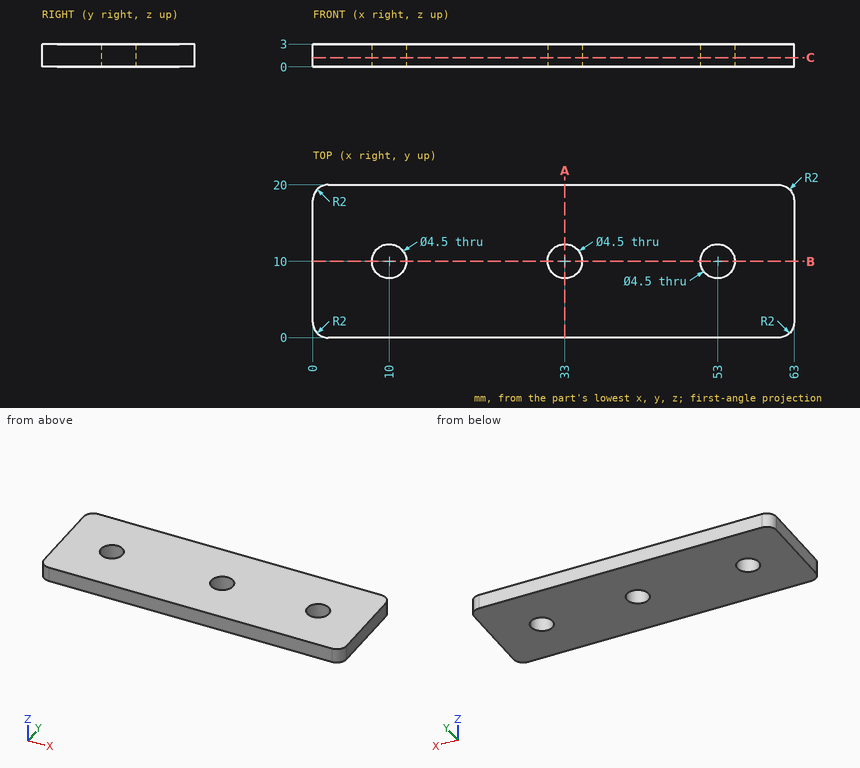
The drawing under review shows one solid part. Ordinate dimensions are in mm from its lowest x, y, z. Give positions to 0.01 mm unless a question says otherwise; leave off trailing zeros. Loops run counter-clockwise (first coordinate to the right, second up) from the corner with the lowest first, then second, coordinate; pieces in that order, holes last. Notation, with made-up numbers: M 42.5,-7.75 L 58.5,-7.75 A30 ccw 58.5,20.25 Z; hole C 55.5,77.25 d11. An arc over 180 degrees is marked long. One line per item, written item: value. Start each with the question number.
Q1. Add section B-B (y = 10). Give the boundary of the cut face in (x, z), and give its area (4 significant figures).
Q2. Add section A-A (x = 33). Give the boundary of the cut face in (y, z).
Q3. Add section C-C (z = 1.2). Give the boundary of the cut face in (x, y), and give its area (3 significant figures).
Q4. For L1, parallel to X at y = 10.25, z = 0.8; L2, parallel to Y at x = 10, z = 0.8; L3, parallel to Y at x = 31, z = 1.1, list the stretches that pass through material, from the lowest coordinate up.
Reply:
1. outline: M 0,0 L 7.75,0 L 7.75,3 L 0,3 Z; M 12.25,0 L 30.75,0 L 30.75,3 L 12.25,3 Z; M 35.25,0 L 50.75,0 L 50.75,3 L 35.25,3 Z; M 55.25,0 L 63,0 L 63,3 L 55.25,3 Z
1. area: 148.5 mm²
2. outline: M 0,0 L 7.75,0 L 7.75,3 L 0,3 Z; M 12.25,0 L 20,0 L 20,3 L 12.25,3 Z
3. outline: M 0,2 A2 ccw 2,0 L 61,0 A2 ccw 63,2 L 63,18 A2 ccw 61,20 L 2,20 A2 ccw 0,18 Z; hole C 10,10 d4.5; hole C 33,10 d4.5; hole C 53,10 d4.5
3. area: 1,210 mm²
4. L1: 0 to 7.76, 12.24 to 30.76, 35.24 to 50.76, 55.24 to 63
4. L2: 0 to 7.75, 12.25 to 20
4. L3: 0 to 8.97, 11.03 to 20
